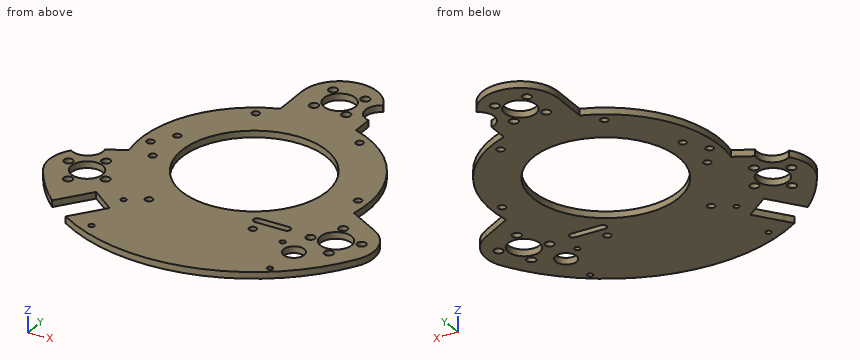
```python
from build123d import *

# Parameters (mm, degrees)
SKETCH1_R           = 2.150000002
SKETCH1_R_2         = 35
SKETCH1_R_3         = 1.8
SKETCH1_R_4         = 7.575
BOSS_EXTRUDE1_DEPTH = 3.175
SKETCH3_R           = 1.35
SKETCH3_R_2         = 5
SKETCH3_W           = 18
SKETCH3_H           = 3.5
CUT_EXTRUDE1_DEPTH  = 3.175
CUT_EXTRUDE2_DEPTH  = 3.175
SKETCH6_R           = 7.5
CUT_EXTRUDE5_DEPTH  = 10
FILLET1_R           = 1.75
SKETCH7_R           = 1.75
CUT_EXTRUDE6_DEPTH  = 10


with BuildPart() as part:
    # Sketch1 → Boss-Extrude1 (new body)
    with BuildSketch(Plane.XY):
        with BuildLine():
            Line((69.097259206, -18.820036388), (54.057762213, -10.136978751))
            ThreePointArc((54.057762213, -10.136978751), (47.631397163, 27.499999965), (18.250000006, 51.883884719))
            Line((18.250000006, 51.883884719), (18.250000006, 69.249999994))
            ThreePointArc((18.250000006, 69.249999994), (6e-09, 87.499999994), (-18.249999994, 69.249999994))
            Line((-18.249999994, 69.249999994), (-18.249999994, 51.883884717))
            ThreePointArc((-18.249999994, 51.883884717), (-47.836716311, 27.141270525), (-53.899300523, -10.948305635))
            Line((-53.899300523, -10.948305635), (-69.097259204, -18.820036383))
            ThreePointArc((-69.097259204, -18.820036383), (-77.600405532, -29.901552426), (-75.777222821, -43.749999994))
            ThreePointArc((-75.777222821, -43.749999994), (0, -87.499999989), (75.777222821, -43.749999994))
            ThreePointArc((75.777222821, -43.749999994), (77.60040553, -29.901552429), (69.097259206, -18.820036388))
        make_face()
        with Locations((-7.778174593, 77.028174587)):
            Circle(SKETCH1_R, mode=Mode.SUBTRACT)
        Circle(SKETCH1_R_2, mode=Mode.SUBTRACT)
        with Locations((-50, 0)):
            Circle(SKETCH1_R_3, mode=Mode.SUBTRACT)
        with Locations((-25, 43.301270189)):
            Circle(SKETCH1_R_3, mode=Mode.SUBTRACT)
        with Locations((25, 43.301270189)):
            Circle(SKETCH1_R_3, mode=Mode.SUBTRACT)
        with Locations((50, 0)):
            Circle(SKETCH1_R_3, mode=Mode.SUBTRACT)
        with Locations((25, -43.301270189)):
            Circle(SKETCH1_R_3, mode=Mode.SUBTRACT)
        with Locations((-25, -43.301270189)):
            Circle(SKETCH1_R_3, mode=Mode.SUBTRACT)
        with Locations((7.778174587, 77.028174593)):
            Circle(SKETCH1_R, mode=Mode.SUBTRACT)
        with Locations((7.778174593, 61.471825413)):
            Circle(SKETCH1_R, mode=Mode.SUBTRACT)
        with Locations((-7.778174587, 61.471825407)):
            Circle(SKETCH1_R, mode=Mode.SUBTRACT)
        with Locations((62.819268711, -45.250184084)):
            Circle(SKETCH1_R, mode=Mode.SUBTRACT)
        with Locations((49.347075128, -37.472009499)):
            Circle(SKETCH1_R, mode=Mode.SUBTRACT)
        with Locations((57.125249713, -23.999815916)):
            Circle(SKETCH1_R, mode=Mode.SUBTRACT)
        with Locations((70.597443296, -31.777990501)):
            Circle(SKETCH1_R, mode=Mode.SUBTRACT)
        with Locations((-70.597443298, -31.777990509)):
            Circle(SKETCH1_R, mode=Mode.SUBTRACT)
        with Locations((-57.125249721, -23.999815914)):
            Circle(SKETCH1_R, mode=Mode.SUBTRACT)
        with Locations((-49.347075126, -37.472009491)):
            Circle(SKETCH1_R, mode=Mode.SUBTRACT)
        with Locations((-62.819268703, -45.250184086)):
            Circle(SKETCH1_R, mode=Mode.SUBTRACT)
        with Locations((0, 69.249999994)):
            Circle(SKETCH1_R_4, mode=Mode.SUBTRACT)
        with Locations((59.972259207, -34.624999997)):
            Circle(SKETCH1_R_4, mode=Mode.SUBTRACT)
        with Locations((-59.972259207, -34.624999997)):
            Circle(SKETCH1_R_4, mode=Mode.SUBTRACT)
    extrude(amount=BOSS_EXTRUDE1_DEPTH)

    # Sketch3 → Cut-Extrude1 (cut)
    with BuildSketch(Plane.XY.offset(3.175)):
        with Locations((-33.85, -49)):
            Circle(SKETCH3_R)
        with Locations((-33.85, -75)):
            Circle(SKETCH3_R)
        with Locations((41.45, -46.7)):
            Circle(SKETCH3_R)
        with Locations((49.972259207, -51.945508073)):
            Circle(SKETCH3_R_2)
        with Locations((48.55, -69)):
            Circle(SKETCH3_R)
        with Locations((30, -36.05)):
            Rectangle(SKETCH3_W, SKETCH3_H)
    extrude(amount=-CUT_EXTRUDE1_DEPTH, mode=Mode.SUBTRACT)

    # Sketch4 → Cut-Extrude2 (cut)
    with BuildSketch(Plane.XY.offset(3.175)):
        Polygon((-18.902035191, 65.231994187), (-24.642286676, 79.090187175), (-38.500479664, 73.349935689), (-32.760228178, 59.491742702), align=None)
        Polygon((-47.04154651, -48.985639752), (-56.172967945, -60.885939856), (-63.507557332, -70.444562845), (-51.607257228, -79.57598428), (-44.272667841, -70.017361292), (-35.141246406, -58.117061187), align=None)
        Polygon((65.943581701, -16.246354435), (80.815254622, -18.204247318), (82.773147505, -3.332574398), (67.901474584, -1.374681515), align=None)
    extrude(amount=-CUT_EXTRUDE2_DEPTH, mode=Mode.SUBTRACT)

    # Sketch6 → Cut-Extrude5 (cut)
    with BuildSketch(Plane.XY):
        with Locations((20, 69.25)):
            Circle(SKETCH6_R)
        with Locations((-69.972259212, -17.304491924)):
            Circle(SKETCH6_R)
    extrude(amount=CUT_EXTRUDE5_DEPTH, mode=Mode.SUBTRACT)

    # Fillet1
    fillet1_edges = [part.edges().sort_by_distance(p)[0] for p in [
        (21, -37.8, 1.5875),
        (39, -37.8, 1.5875),
        (39, -34.3, 1.5875),
        (21, -34.3, 1.5875),
    ]]
    fillet(fillet1_edges, radius=FILLET1_R - 0.0001)  # a hair under: the kernel refuses the full size

    # Sketch7 → Cut-Extrude6 (cut)
    with BuildSketch(Plane.XY.offset(3.175)):
        with Locations((-43, 10)):
            Circle(SKETCH7_R)
        with Locations((-43, -10)):
            Circle(SKETCH7_R)
    extrude(amount=-CUT_EXTRUDE6_DEPTH, mode=Mode.SUBTRACT)


solid = part.part
```
Here's how the part is built. I have some questions about the finished solid (model axes, mm). Give positions to 0.01 mm unless a question says otherwise; leave off trailing zeros. Write each loop counter-clockwise with the first axis right and the second up, starting at its lowest first coordinate (ties: lowest second). Pieces come first, ordered by that corner, then holes.
(1) Imagine slicing it at A-A, the plane x = 0. Write out the boundary of the cut face in (y, z) (3 decimals).
Output values:
outline: (-87.5, 0) - (-35, 0) - (-35, 3.175) - (-87.5, 3.175) - close; (35, 0) - (61.675, 0) - (61.675, 3.175) - (35, 3.175) - close; (76.825, 0) - (87.5, 0) - (87.5, 3.175) - (76.825, 3.175) - close
(2) If I drill on L1, parallel to Y at x = 0, z = 1.3 (3 decimals); L2, parallel to Y at x = 58, z = 2.7; L3, parallel to Y at x = -70.5, z = 2, over which ranges is the centre line in solid material (lowest first)?
Output values:
L1: y = -87.5 to -35, 35 to 61.675, 76.825 to 87.5
L2: y = -65.52 to -41.94, -27.31 to -25.96, -22.04 to -12.41
L3: y = -51.83 to -33.93, -29.63 to -24.79
(3) Imagine slicing it at C-C, the plane y = 55.5. Write out the boundary of the cut face in (x, z) (3 decimals), and give its area (3 significant figures).
Output values:
outline: (-18.25, 0) - (18.25, 0) - (18.25, 3.175) - (-18.25, 3.175) - close
area: 116 mm2
(4) Will these pins go through, and if not, where does the flat tip stop? pin 1 (1 mm diameter, centred on y = -66, z = 1, fed in from -X); pin 2 (1.5 mm diameter, centred on y = -2.5, z = 1, fed in from -X); pin 3 (1 mm diameter, centred on y = 51.5, z = 1, fed in from +X).
Output values:
pin 1: stops at x = -41.57
pin 2: stops at x = -54.97
pin 3: stops at x = 20.59
(5) Imagine slicing it at B-B, the plane y = 14. Write out the boundary of the cut face in (x, z) (3 decimals), and give its area (3 significant figures).
Output values:
outline: (-53.188, 0) - (-32.078, 0) - (-32.078, 3.175) - (-53.188, 3.175) - close; (32.078, 0) - (53.188, 0) - (53.188, 3.175) - (32.078, 3.175) - close
area: 134 mm2
